Design review of the part built by this model. Coordinates are the model's own, in mm. Face numbers are marked on the shaded views. A direction names the side the tool comes from. Coordinates: 2 decimals unless noted, no trailing zeros. Write each loop counter-clockwise with the first axis right and the second up, starting at its lowest first coordinate (ties: lowest second). Pieces come first, ordered by that corner, then holes. Notation, with made-up numbers: (45, 73) -> (54, 73) arc R19 ccw to (54, 85) -> close; hole circle Ø11 at (83, -39.5). An arc over 180 degrees is marked (long way). Return JSON: item names as keys, results as strings. Group by question number.
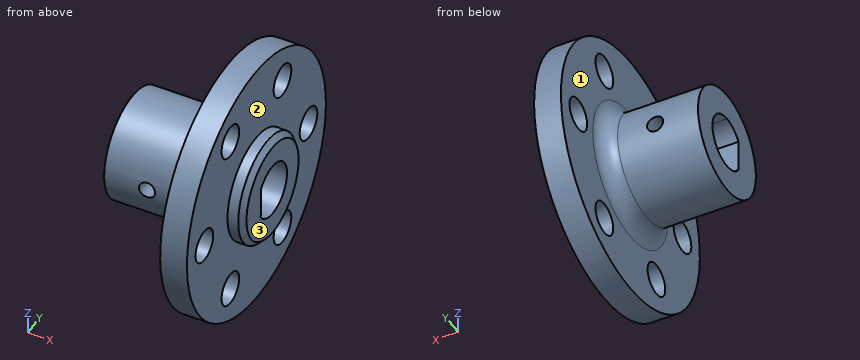
from build123d import *

# Parameters (mm, degrees)
SKETCH_1_R               = 24
SKETCH_1_R_2             = 3.05
EXTRUDE_1_DEPTH          = 5
SKETCH_14_R              = 10
EXTRUDE_2_DEPTH          = 3
SKETCH_15_R              = 10
EXTRUDE_3_DEPTH          = 18
CUT_EXTRUDE_1_DEPTH      = 27
FILLET_5_R               = 3
CHAMFER_1_SIZE           = 1
SKETCH_18_R              = 1.5
CUT_EXTRUDE_4_DEPTH      = 29.344105586
CUT_EXTRUDE_4_DEPTH_BACK = 21.267784004


with BuildPart() as part:
    # Sketch 1 → 凸台-拉伸1 (new body)
    with BuildSketch(Plane(origin=(0, 0, 0), x_dir=(0, 0, -1), z_dir=(1, 0, 0))):
        Circle(SKETCH_1_R)
        with Locations((-15.588457268, 9)):
            Circle(SKETCH_1_R_2, mode=Mode.SUBTRACT)
        with Locations((0, 18)):
            Circle(SKETCH_1_R_2, mode=Mode.SUBTRACT)
        with Locations((15.588457268, 9)):
            Circle(SKETCH_1_R_2, mode=Mode.SUBTRACT)
        with Locations((15.588457268, -9)):
            Circle(SKETCH_1_R_2, mode=Mode.SUBTRACT)
        with Locations((0, -18)):
            Circle(SKETCH_1_R_2, mode=Mode.SUBTRACT)
        with Locations((-15.588457268, -9)):
            Circle(SKETCH_1_R_2, mode=Mode.SUBTRACT)
    extrude(amount=EXTRUDE_1_DEPTH)

    # 草图14 → 凸台-拉伸2 (add)
    with BuildSketch(Plane(origin=(5, 0, 0), x_dir=(0, 0, -1), z_dir=(1, 0, 0))):
        Circle(SKETCH_14_R)
    extrude(amount=EXTRUDE_2_DEPTH)

    # 草图15 → 凸台-拉伸3 (add)
    with BuildSketch(Plane.ZY):
        Circle(SKETCH_15_R)
    extrude(amount=EXTRUDE_3_DEPTH)

    # 草图16 → 切除-拉伸1 (cut, through all)
    with BuildSketch(Plane.ZY.offset(18)):
        with BuildLine():
            ThreePointArc((5, 0), (-2.29326147, 4.443079093), (-2.896380732, -4.075656838))
            Line((-2.896380732, -4.075656838), (3, -4))
            ThreePointArc((3, -4), (4.472135955, -2.236067977), (5, 0))
        make_face()
    extrude(amount=-CUT_EXTRUDE_1_DEPTH, mode=Mode.SUBTRACT)

    # 圆角5
    fillet_5_edges = [part.edges().sort_by_distance(p)[0] for p in [
        (0, 0, -10),
    ]]
    fillet(fillet_5_edges, radius=FILLET_5_R)

    # 倒角1
    chamfer_1_edges = [part.edges().sort_by_distance(p)[0] for p in [
        (8, 0, 10),
    ]]
    chamfer(chamfer_1_edges, length=CHAMFER_1_SIZE)

    # 草图18 → 切除-拉伸4 (cut, two sides)
    with BuildSketch(Plane(origin=(0, -4.037828419, 0.051809634), x_dir=(1, 0, 0), z_dir=(0, 0.999917692, -0.012830008))) as cut_extrude_4_sk:
        with Locations((-10, 0)):
            Circle(SKETCH_18_R)
    extrude(amount=CUT_EXTRUDE_4_DEPTH, mode=Mode.SUBTRACT)
    extrude(cut_extrude_4_sk.sketch, amount=-CUT_EXTRUDE_4_DEPTH_BACK, mode=Mode.SUBTRACT)


solid = part.part
Q1. For the marked faces 1, 2 and 3, list the 3-axis set-ups (+Z, -Z, +X, -X, +Y, -Y) from which the entire face can be reached by the end or side of a thin tool; tool diameter is ignored.
Q2. We need section C-C on x = -15. Write out the cut boundary in (y, z), plus the area to 3 significant figures.
Q3. We need section B-B on y = -18. Write out the cut boundary in (x, z).
Q4. For P1, Ø10, axis at x = 0.5, z = 10.5, coming from the +Y side; P2, Ø1.5, axis at x = -1, y = 12.5, coming from the -Z side (3 decimals); P3, Ø4, axis at y = 9.5, z = -12, coming from the +X side; P4, Ø8, axis at y = 16, z = 17, coming from the -X side, all flat-tipped, find the tip position at first contact; note any pin that passes through.
Q5. Wall thickness on L1, parallel to Y at x = 3, z = -2; L2, parallel to Y at x = 1.25, z = 0; L3, parallel to X at y = -15, z = 17.5: over which ranges is each line inside the solid? List them lowest first.
Q6. We need section A-A on z = 15. Write out the cut boundary in (x, y) (3 decimals).
Findings below:
{
 "1": {"face 1": "-X", "face 2": "+X", "face 3": "+Z, -Z, +X, +Y, -Y"},
 "2": {"outline": "circle Ø20 at (0, 0); hole (-4.08, -2.9) arc R5 ccw (long way) to (-4, 3) -> close", "area": "239 mm^2"},
 "3": {"outline": "(0, -15.87) -> (5, -15.87) -> (5, -3.05) -> (0, -3.05) -> close; (0, 3.05) -> (5, 3.05) -> (5, 15.87) -> (0, 15.87) -> close"},
 "4": {"P1": "stops at y = 23.36", "P2": "passes through", "P3": "stops at x = 5", "P4": "stops at x = 0"},
 "5": {"L1": "y = -23.92 to -20.3, -15.7 to -4.06, 4.58 to 15.7, 20.3 to 23.92", "L2": "y = -24 to -21.05, -14.95 to -4.04, 5 to 14.95, 21.05 to 24", "L3": "x = 0 to 5"},
 "6": {"outline": "(0, -18.735) -> (5, -18.735) -> (5, -11.993) -> (0, -11.993) -> close; (0, -6.007) -> (5, -6.007) -> (5, 6.007) -> (0, 6.007) -> close; (0, 11.993) -> (5, 11.993) -> (5, 18.735) -> (0, 18.735) -> close"}
}
